```python
from build123d import *

# Parameters (mm, degrees)
SKETCH1_W           = 20
SKETCH1_H           = 15
BOSS_EXTRUDE1_DEPTH = 3.5
BOSS_EXTRUDE8_DEPTH = 1.5
SKETCH3_W           = 3.4
SKETCH3_H           = 1
CUT_EXTRUDE1_DEPTH  = 18.642278764
SKETCH7_R           = 1.25
CUT_EXTRUDE4_DEPTH  = 17.650825805
SKETCH8_W           = 10
SKETCH8_H           = 7
BOSS_EXTRUDE9_DEPTH = 4
CUT_EXTRUDE5_DEPTH  = 0.5
SKETCH10_W          = 8
SKETCH10_H          = 3.5
CUT_EXTRUDE6_DEPTH  = 21.856653615


with BuildPart() as part:
    # Sketch1 → Boss-Extrude1 (new body)
    with BuildSketch(Plane.XY):
        Rectangle(SKETCH1_W, SKETCH1_H)
    extrude(amount=BOSS_EXTRUDE1_DEPTH)

    # Sketch2 → Boss-Extrude8 (add)
    with BuildSketch(Plane.XY.offset(3.5)):
        Polygon((-6.431580724, 2), (-10, 2), (-10, 1.5), (-10, 0.3), (-10, -2), (-6.431580724, -2), (-6.431580724, -1.5), (-9.8, -1.5), (-9.8, -0.2), (-6.431580724, -0.2), (-6.431580724, 0.3), (-9.8, 0.3), (-9.8, 1.5), (-6.431580724, 1.5), align=None)
        Polygon((-10, 1.5), (-10, 2), (-14, 2), (-14, -2), (-10, -2), (-10, 0.3), align=None)
    extrude(amount=BOSS_EXTRUDE8_DEPTH)

    # Sketch3 → Cut-Extrude1 (cut, through all)
    with BuildSketch(Plane.XZ.offset(2)):
        with Locations((-8.631580724, 4)):
            Rectangle(SKETCH3_W, SKETCH3_H)
    extrude(amount=-CUT_EXTRUDE1_DEPTH, mode=Mode.SUBTRACT)

    # Sketch7 → Cut-Extrude4 (cut, through all)
    with BuildSketch(Plane(origin=(0, 0, 0), x_dir=(-1, 0, 0), z_dir=(0, 0, -1))):
        with Locations((8, -5)):
            Circle(SKETCH7_R)
        with Locations((8, 5)):
            Circle(SKETCH7_R)
    extrude(amount=-CUT_EXTRUDE4_DEPTH, mode=Mode.SUBTRACT)

    # Sketch8 → Boss-Extrude9 (add)
    with BuildSketch(Plane(origin=(0, 0, 0), x_dir=(-1, 0, 0), z_dir=(0, 0, -1))):
        with Locations((-12, 0)):
            Rectangle(SKETCH8_W, SKETCH8_H)
    extrude(amount=BOSS_EXTRUDE9_DEPTH)

    # Sketch9 → Cut-Extrude5 (cut)
    with BuildSketch(Plane(origin=(0, 0, -4), x_dir=(-1, 0, 0), z_dir=(0, 0, -1))):
        Polygon((-6, -3), (-18, -3), (-18, 3), (-6, 3), (-6, 0.25), (-16.368004225, 0.25), (-16.368004225, -0.25), (-6, -0.25), align=None)
    extrude(amount=-CUT_EXTRUDE5_DEPTH, mode=Mode.SUBTRACT)

    # Sketch10 → Cut-Extrude6 (cut, through all)
    with BuildSketch(Plane(origin=(0, 3.5, 0), x_dir=(1, 0, 0), z_dir=(0, 1, 0))):
        with Locations((13, 1.75)):
            Rectangle(SKETCH10_W, SKETCH10_H)
    extrude(amount=-CUT_EXTRUDE6_DEPTH, mode=Mode.SUBTRACT)


solid = part.part
```
The model under review builds one solid part; all positions refer to its coordinate system, in mm. A direction names the side the tool comes from. Give positions to 0.01 mm unless a question says otherwise; leave off trailing zeros. Write each loop counter-clockwise with the first axis right and the second up, starting at its lowest first coordinate (ties: lowest second). Pieces come first, ordered by that corner, then holes.
(1) To check wall thickness, follow L1, parallel to Y at x = -8, z = 1.4; L2, parallel to X at y = 2, z = -1; L3, parallel to X at y = 6.5, z = 1.25. State the ranges of each line that lie inside material, in increasing order.
(2) Consider section B-B, the plane x = 14.5. Give the boundary of the cut face in (y, z), and give its area (3 significant figures).
(3) For P1, Ø1.5, axis at y = -1, z = -1.5, coming from the +X side; P2, Ø7.5, axis at x = -5, y = -2.5, coming from the -Z side; P3, Ø0.6, axis at y = 0, z = 4.5, coming from the +X side, all flat-tipped, find the tip position at first contact; note any pin that passes through.
(4) Consider section A-A, the plane y = -5. Give the boundary of the cut face in (x, z), and give its area (4 significant figures).
(5) Consider section D-D, the plane z = 1. Give the boundary of the cut face in (x, y).
(6) The part is to be moulded in two halves that separate along Z. For faces 1 (the flat face through (9, 0, -2)), 2 (the flat face through (-11, 0, 5)), 3 (the flat face through (-9, 0, 4.5)), 4 (the flat face through (-7.7, 0.3, 4.7)), say which applies: released by +Z, released by -Z, zero draft, split by the parting line, or undercut.
(7) Tool access review of faces 5 (the flat face through (-11, 2, 4)), 6 (the flat face through (10, 0, 2)), 7 (the flat face through (-7.7, -1.5, 4.7)): name each direction out of +Z, -Z, +X, -X, +Y, -Y from which nothing blocks a thin tool from reaching the whole face with its end or side.
(8) Consider section C-C, the plane x = -8. Give the boundary of the cut face in (y, z).
Returned:
1. L1: y = -7.5 to -6.25, -3.75 to 3.75, 6.25 to 7.5
1. L2: x = 7 to 9
1. L3: x = -10 to 10
2. outline: (-3.5, -4) - (-3, -4) - (-3, -3.5) - (-3.5, -3.5) - close; (-0.25, -4) - (0.25, -4) - (0.25, -3.5) - (-0.25, -3.5) - close; (3, -4) - (3.5, -4) - (3.5, -3.5) - (3, -3.5) - close
2. area: 0.750 mm2
3. P1: stops at x = 9
3. P2: stops at z = 0
3. P3: stops at x = -6.43
4. outline: (-10, 0) - (-9.25, 0) - (-9.25, 3.5) - (-10, 3.5) - close; (-6.75, 0) - (10, 0) - (10, 3.5) - (-6.75, 3.5) - close
4. area: 61.25 mm2
5. outline: (-10, -7.5) - (10, -7.5) - (10, 7.5) - (-10, 7.5) - close; hole circle Ø2.5 at (-8, -5); hole circle Ø2.5 at (-8, 5)
6. face 1: undercut
6. face 2: released by +Z
6. face 3: undercut
6. face 4: zero draft
7. face 5: +Z, +X, -X, +Y
7. face 6: +Z, +X, +Y, -Y
7. face 7: +Z, +X
8. outline: (-7.5, 0) - (-6.25, 0) - (-6.25, 3.5) - (-7.5, 3.5) - close; (-3.75, 0) - (3.75, 0) - (3.75, 3.5) - (-3.75, 3.5) - close; (-2, 4.5) - (-1.5, 4.5) - (-1.5, 5) - (-2, 5) - close; (-0.2, 4.5) - (0.3, 4.5) - (0.3, 5) - (-0.2, 5) - close; (1.5, 4.5) - (2, 4.5) - (2, 5) - (1.5, 5) - close; (6.25, 0) - (7.5, 0) - (7.5, 3.5) - (6.25, 3.5) - close
